Read the model definition and answer for the solid it produces. Units are mm, in the model's axes. Face numbers are marked on the shaded views. A direction names the side the tool comes from. Coordinates: 2 decimals unless noted, no trailing zeros. Write each loop counter-clockwise with the first axis right and the second up, starting at its lowest first coordinate (ties: lowest second). Pieces come first, ordered by that corner, then holes. Notation, with made-up numbers: (12, 55) -> (40, 55) arc R23 ccw to (40, 68) -> close; hole circle Ø2 at (10, -3). An arc over 180 degrees is marked (long way). Use CSV: the item, a comma, the result in double quotes. Start each with the question number.
from build123d import *

# Parameters (mm, degrees)
F0_W     = 50.8
F0_H     = 19.05
F1_DEPTH = 749.3
F2_W     = 122.435573
F2_H     = 50.8
F2_W_2   = 93.867282
F2_W_3   = 343.160421
F2_H_2   = 127
F3_DEPTH = 25.4
F4_R     = 0.79375
F5_DEPTH = 25.4


with BuildPart() as f1:
    # F0 (on Top) → F1 (new body)
    with BuildSketch(Plane.XY):
        Rectangle(F0_W, F0_H)
    extrude(amount=F1_DEPTH)

    # F2 (on Front) → F3 (cut)
    with BuildSketch(Plane.XZ):
        with Locations((22.446524, 25.4)):
            Rectangle(F2_W, F2_H)
        with Locations((2.720783, 393.7)):
            Rectangle(F2_W_2, F2_H)
        with Locations((-38.781822, 685.8)):
            Rectangle(F2_W_3, F2_H_2)
    extrude(amount=F3_DEPTH, mode=Mode.SUBTRACT)

    # F4 (on Front) → F5 (cut)
    with BuildSketch(Plane.XZ):
        with Locations((9.525, 101.6)):
            Circle(F4_R)
        with Locations((9.525, 155.575)):
            Circle(F4_R)
        with Locations((9.525, 263.525)):
            Circle(F4_R)
        with Locations((9.525, 317.5)):
            Circle(F4_R)
        with Locations((-9.525, 263.525)):
            Circle(F4_R)
        with Locations((-9.525, 317.5)):
            Circle(F4_R)
        with Locations((-9.525, 101.6)):
            Circle(F4_R)
        with Locations((-9.525, 155.575)):
            Circle(F4_R)
    extrude(amount=-F5_DEPTH, mode=Mode.SUBTRACT)


solid = f1.part
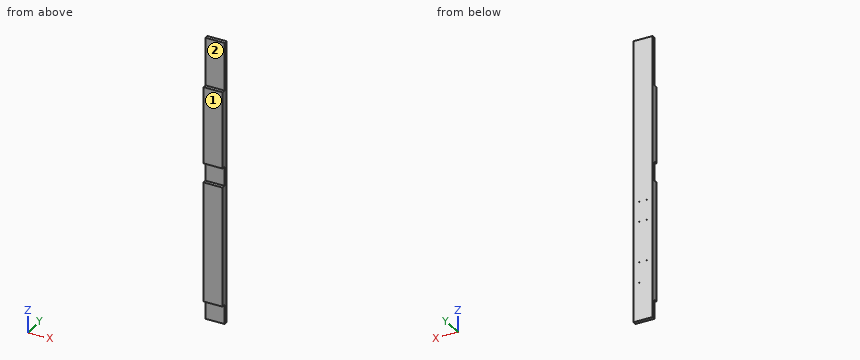
1) Section C-C, the plane z = 391.5 is taken. Give the vertices of the cut face in (x, y) (3 decimals), plus the area to 3 significant figures.
2) Section A-A, the plane y = -4.5 is taken. Give the vertices of the cut face in (x, z), plus the area to 3 significant figures.
3) Section B-B, the plane x = 18 is taken. Give the vertices of the cut face in (y, z) (3 decimals).
4) Find the intervals of material crossed by line 1 along X through (y, z) = (6, 317.5); line 2 along Z through (x, y) = (6, -7.5); line 3 along Y through (x, z) = (20, 687) (3 decimals), in increasing order.
5) Each of these flat-tipped pins is pushed along its axis until it touches: pin 1 (3 mm diameter, centred on x = -19, y = -2, fed in from -Z); pin 2 (1.3 mm diameter, centred on x = -9.5, z = 317.5, fed in from +Y); pin 3 (10.5 mm diameter, centred on x = -4, y = -6, fed in from +Z). Where does it stop, or does it pass through?
6) Which of the six approach directions +Z, -Z, +X, -X, +Y, -Y give full straight-line access (tool end or side, diameter ignored) to the marked faces 1 and 2?
The answers:
1,outline,"(-25.4, 0) -> (25.4, 0) -> (25.4, 9.525) -> (-25.4, 9.525) -> close"
1,area,"484 mm^2"
2,outline,"(-25.4, 50.8) -> (25.4, 50.8) -> (25.4, 368.3) -> (-25.4, 368.3) -> close; (-25.4, 419.1) -> (25.4, 419.1) -> (25.4, 622.3) -> (-25.4, 622.3) -> close"
2,area,"26,500 mm^2"
3,outline,"(-9.525, 50.8) -> (0, 50.8) -> (0, 0) -> (9.525, 0) -> (9.525, 749.3) -> (0, 749.3) -> (0, 622.3) -> (-9.525, 622.3) -> (-9.525, 419.1) -> (0, 419.1) -> (0, 368.3) -> (-9.525, 368.3) -> close"
4,line 1,"x = -25.4 to -10.32, -8.73 to 8.73, 10.32 to 25.4"
4,line 2,"z = 50.8 to 368.3, 419.1 to 622.3"
4,line 3,"y = 0 to 9.525"
5,pin 1,"stops at z = 50.8"
5,pin 2,"stops at y = 0"
5,pin 3,"stops at z = 622.3"
6,face 1,"+Z, -Z, +X, -X, -Y"
6,face 2,"+Z, +X, -X, -Y"
